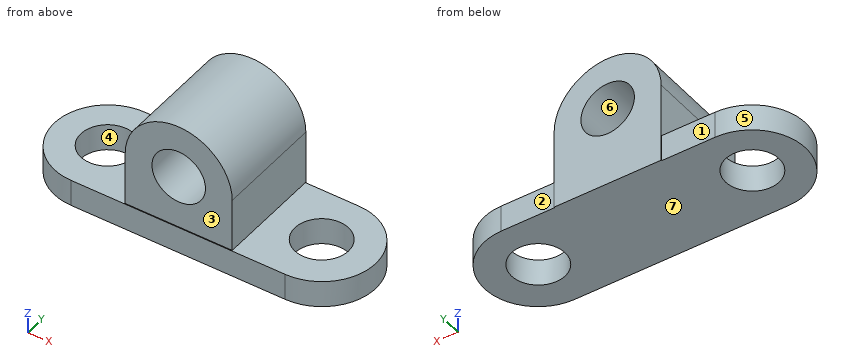
Autodesk Fusion 360 part; units mm, degrees
sketch "Sketch1" plane through (0, 0, 0) normal (0, 0, 1) x (1, 0, 0)
  line L0 (40.3277, 19.712) -> (-39.6723, 19.712)
  line L1 (-39.6723, 19.712) -> (-39.6723, -20.288)
  line L2 (-39.6723, -20.288) -> (40.3277, -20.288)
  line L3 (40.3277, -20.288) -> (40.3277, 19.712)
  line L4 (-39.6723, -0.288) -> (40.3277, -0.288) construction
  circle A0 centre (40, 0) radius 10
  circle A1 centre (-40, 0) radius 10
  line L5 (-24, 12) -> (-20, 10) construction
  line L6 (24, 12) -> (20, 10) construction
  arc A2 (40.3277, -20.288) -> (40.3277, 19.712) centre (40.3277, -0.288) ccw
  arc A3 (-39.6723, 19.712) -> (-39.6723, -20.288) centre (-39.6723, -0.288) ccw
  dimension "d1" = 80
  dimension "d2" = 40
  dimension "d6" = 40
  dimension "d7" = 40
sketch "Sketch2" plane through (0, 0, 0) normal (0, 0, 1) x (1, 0, 0)
sketch "Sketch3" plane through (0, 0, 0) normal (0, 0, 1) x (1, 0, 0)
extrude "Extrude1" add sketch "Sketch1" along normal blind 10 contours L0 L1 L2 L3 A0 A1 | L3 A0 A2 | L1 A1 A3
sketch "Sketch4" plane through (0, 0, 0) normal (0, 1, 0) x (1, 0, 0)
  line L0 (-19.6723, 0) -> (20.3277, 0)
  line L1 (20.3277, 0) -> (20.3277, -30)
  line L2 (-19.6723, -30) -> (-19.6723, 0)
  line L3 (-39.6723, 0) -> (-39.6723, -10)
  circle A0 centre (0.3277, -30) radius 10
  arc A1 (-19.6723, -30) -> (20.3277, -30) centre (0.3277, -30) ccw
  dimension "d12" = 30
  dimension "d13" = 40
  dimension "d14" = 20
  dimension "d15" = 40
  dimension "d16" = 20
extrude "Extrude2" add sketch "Sketch4" along normal mid plane 40
Source: CAD feature listing. Evaluate the final solid. Frame: model axes, mm. Face numbers are marked on the shaded views. A direction names the side the tool comes from. Give positions to 0.01 mm unless a question says otherwise; leave off trailing zeros. Order: outer loops, then holes, each group sorted by start corner. A loop starts at its lowest first (then second) coordinate and runs counter-clockwise, first axis right, second up. Notation, with made-up numbers: (-11.5, 9) -> (17.5, 9) arc R22 cw to (17.5, 45) -> close; hole circle Ø10 at (58, 2). An arc over 180 degrees is marked (long way). Write item = value, one per line.
Q1. Material intervals for line 1 (X direction, y = 0, z = 3.5); line 2 (Y direction, x = -40, z = 4); line 3 (X direction, y = 10.5, z = 30), sorted ascending. Write a range as from..to.
Data:
line_1 = -59.67..-50, -30..30, 50..60.33
line_2 = -20.29..-10, 10..19.71
line_3 = -19.67..-9.67, 10.33..20.33
Q2. Cut plane A-A, the plane y = 0. Output: boundary loops of the cut face in (x, z), and give its area (3 significant figures).
Data:
outline = (-59.67, 0) -> (-50, 0) -> (-50, 10) -> (-59.67, 10) -> close; (-30, 0) -> (30, 0) -> (30, 10) -> (20.33, 10) -> (20.33, 30) arc R20 ccw to (-19.67, 30) -> (-19.67, 10) -> (-30, 10) -> close; (50, 0) -> (60.33, 0) -> (60.33, 10) -> (50, 10) -> close; hole circle Ø20 at (0.33, 30)
area = 1,910 mm^2
Q3. Cut plane B-B, the plane x = 48. Output: boundary loops of the cut face in (y, z).
Data:
outline = (-18.76, 0) -> (-6, 0) -> (-6, 10) -> (-18.76, 10) -> close; (6, 0) -> (18.18, 0) -> (18.18, 10) -> (6, 10) -> close
Q4. Pull-direction query (X, two-part tool) for the marked faces 4, 5, 6 and 7; classes: released by +X, released by -X, zero draft, split by the parting line, or undercut.
Data:
face_4 = undercut
face_5 = released by -X
face_6 = undercut
face_7 = zero draft
Q5. Pin query (flat end, axial travel): pin 1 (24 mm diameter, centred on y = 3.5, z = 18.5, fed in from -X); pin 2 (1.5 mm diameter, centred on x = 21.5, y = 14.5, fed in from +Z); pin 3 (8 mm diameter, centred on x = 35, z = 5.5, fed in from +Y); pin 4 (12 mm diameter, centred on x = 40, y = 0, fed in from +Z). Return the tip coordinate at first contact, or that it passes through.
Data:
pin_1 = -59.67
pin_2 = 10
pin_3 = 19.71
pin_4 = through
Q6. Set-up query: the marked faces 1, 2 and 3. Return all of +Z, -Z, +X, -X, +Y, -Y with unobstructed straight access to the full face (end or side cutting, diameter ignored); none if empty.
Data:
face_1 = +Z, -Z, -X, +Y
face_2 = +Z, -Z, +X, +Y
face_3 = +Z, +X, -X, -Y
Q7. Cut plane C-C, the plane y = -5. Output: boundary loops of the cut face in (x, z), and give its area (3 significant figures).
Data:
outline = (-59.11, 0) -> (-48.66, 0) -> (-48.66, 10) -> (-59.11, 10) -> close; (-31.34, 0) -> (31.34, 0) -> (31.34, 10) -> (20.33, 10) -> (20.33, 30) arc R20 ccw to (-19.67, 30) -> (-19.67, 10) -> (-31.34, 10) -> close; (48.66, 0) -> (59.76, 0) -> (59.76, 10) -> (48.66, 10) -> close; hole circle Ø20 at (0.33, 30)
area = 1,960 mm^2
Q8. Cut plane D-D, the plane z = 33.5. Output: boundary loops of the cut face in (x, y), and give its area (3 significant figures).
Data:
outline = (-19.36, -20) -> (-9.04, -20) -> (-9.04, 20) -> (-19.36, 20) -> close; (9.7, -20) -> (20.02, -20) -> (20.02, 20) -> (9.7, 20) -> close
area = 826 mm^2
